For this review, take the finished solid that the model builds, in its own axes (mm). A direction names the side the tool comes from. Give positions to 0.01 mm unless a question says otherwise; leave off trailing zeros. Loops run counter-clockwise (first coordinate to the right, second up) from the corner with the lowest first, then second, coordinate; pieces in that order, holes last. Notation, with made-up numbers: (10, 55) - (18, 55) arc R30 ccw to (18, 83) - close; hole circle Ø3 at (45.25, -26.5). An arc over 180 degrees is marked (long way). Answer as CSV lines item,"result".
from build123d import *

# Parameters (mm, degrees)
SKETCH1_W           = 130
SKETCH1_H           = 50
BOSS_EXTRUDE1_DEPTH = 5
SKETCH2_W           = 130
SKETCH2_H           = 5
BOSS_EXTRUDE2_DEPTH = 32
SKETCH3_R           = 3
SKETCH3_W           = 5
SKETCH3_H           = 10
CUT_EXTRUDE1_DEPTH  = 10
FILLET1_R           = 5
CUT_EXTRUDE2_REACH  = 88.597
SKETCH4_R           = 3.15
SKETCH4_R_2         = 2.15


with BuildPart() as part:
    # Sketch1 → Boss-Extrude1 (new body)
    with BuildSketch(Plane(origin=(0, 0, 0), x_dir=(1, 0, 0), z_dir=(0, 1, 0))):
        Rectangle(SKETCH1_W, SKETCH1_H)
    extrude(amount=BOSS_EXTRUDE1_DEPTH)

    # Sketch2 → Boss-Extrude2 (add)
    with BuildSketch(Plane(origin=(0, 0, -25), x_dir=(-1, 0, 0), z_dir=(0, 0, -1))):
        with Locations((0, 2.5)):
            Rectangle(SKETCH2_W, SKETCH2_H)
    extrude(amount=BOSS_EXTRUDE2_DEPTH)

    # Sketch3 → Cut-Extrude1 (cut)
    with BuildSketch(Plane(origin=(0, 5, 0), x_dir=(1, 0, 0), z_dir=(0, 1, 0))):
        with Locations(Location((-57.5, 31.5, 0), (0, 0, 270))):
            Circle(SKETCH3_R)
        with Locations(Location((57.5, 31.5, 0), (0, 0, 270))):
            Circle(SKETCH3_R)
        with Locations((57.5, 44)):
            Rectangle(SKETCH3_W, SKETCH3_H)
        with Locations((-57.5, 19)):
            Rectangle(SKETCH3_W, SKETCH3_H)
        with Locations((-57.5, 44)):
            Rectangle(SKETCH3_W, SKETCH3_H)
        with Locations((57.5, 19)):
            Rectangle(SKETCH3_W, SKETCH3_H)
    extrude(amount=-CUT_EXTRUDE1_DEPTH, mode=Mode.SUBTRACT)

    # Fillet1
    fillet1_edges = [part.edges().sort_by_distance(p)[0] for p in [
        (65, 2.5, -57),
        (-65, 2.5, -57),
        (65, 2.5, 25),
        (-65, 2.5, 25),
    ]]
    fillet(fillet1_edges, radius=FILLET1_R)

    # Sketch4 → Cut-Extrude2 (cut, up to next)
    with BuildSketch(Plane(origin=(0, 5, 0), x_dir=(1, 0, 0), z_dir=(0, 1, 0)), mode=Mode.PRIVATE) as cut_extrude2_sk1:
        with Locations(Location((0, -0.5, 0), (0, 0, 270))):
            Circle(SKETCH4_R)
    cut_extrude2_tool1 = extrude(cut_extrude2_sk1.sketch, amount=-CUT_EXTRUDE2_REACH, mode=Mode.PRIVATE) & part.part
    # Sketch4 → Cut-Extrude2 (cut, up to next)
    with BuildSketch(Plane(origin=(0, 5, 0), x_dir=(1, 0, 0), z_dir=(0, 1, 0)), mode=Mode.PRIVATE) as cut_extrude2_sk2:
        with Locations(Location((25.4, 43.55, 0), (0, 0, 270))):
            Circle(SKETCH4_R_2)
    cut_extrude2_tool2 = extrude(cut_extrude2_sk2.sketch, amount=-CUT_EXTRUDE2_REACH, mode=Mode.PRIVATE) & part.part
    # Sketch4 → Cut-Extrude2 (cut, up to next)
    with BuildSketch(Plane(origin=(0, 5, 0), x_dir=(1, 0, 0), z_dir=(0, 1, 0)), mode=Mode.PRIVATE) as cut_extrude2_sk3:
        with Locations(Location((-25.4, 43.55, 0), (0, 0, 270))):
            Circle(SKETCH4_R_2)
    cut_extrude2_tool3 = extrude(cut_extrude2_sk3.sketch, amount=-CUT_EXTRUDE2_REACH, mode=Mode.PRIVATE) & part.part
    # Sketch4 → Cut-Extrude2 (cut, up to next)
    with BuildSketch(Plane(origin=(0, 5, 0), x_dir=(1, 0, 0), z_dir=(0, 1, 0)), mode=Mode.PRIVATE) as cut_extrude2_sk4:
        with Locations(Location((-12.7, 43.55, 0), (0, 0, 270))):
            Circle(SKETCH4_R_2)
    cut_extrude2_tool4 = extrude(cut_extrude2_sk4.sketch, amount=-CUT_EXTRUDE2_REACH, mode=Mode.PRIVATE) & part.part
    # Sketch4 → Cut-Extrude2 (cut, up to next)
    with BuildSketch(Plane(origin=(0, 5, 0), x_dir=(1, 0, 0), z_dir=(0, 1, 0)), mode=Mode.PRIVATE) as cut_extrude2_sk5:
        with Locations(Location((12.7, 43.55, 0), (0, 0, 270))):
            Circle(SKETCH4_R_2)
    cut_extrude2_tool5 = extrude(cut_extrude2_sk5.sketch, amount=-CUT_EXTRUDE2_REACH, mode=Mode.PRIVATE) & part.part
    # Sketch4 → Cut-Extrude2 (cut, up to next)
    with BuildSketch(Plane(origin=(0, 5, 0), x_dir=(1, 0, 0), z_dir=(0, 1, 0)), mode=Mode.PRIVATE) as cut_extrude2_sk6:
        with Locations(Location((0, 43.55, 0), (0, 0, 270))):
            Circle(SKETCH4_R_2)
    cut_extrude2_tool6 = extrude(cut_extrude2_sk6.sketch, amount=-CUT_EXTRUDE2_REACH, mode=Mode.PRIVATE) & part.part
    add(cut_extrude2_tool1.solids().sort_by_distance((0, 5, 0.5))[0], mode=Mode.SUBTRACT)
    add(cut_extrude2_tool2.solids().sort_by_distance((25.4, 5, -43.55))[0], mode=Mode.SUBTRACT)
    add(cut_extrude2_tool3.solids().sort_by_distance((-25.4, 5, -43.55))[0], mode=Mode.SUBTRACT)
    add(cut_extrude2_tool4.solids().sort_by_distance((-12.7, 5, -43.55))[0], mode=Mode.SUBTRACT)
    add(cut_extrude2_tool5.solids().sort_by_distance((12.7, 5, -43.55))[0], mode=Mode.SUBTRACT)
    add(cut_extrude2_tool6.solids().sort_by_distance((0, 5, -43.55))[0], mode=Mode.SUBTRACT)


solid = part.part
1) Insertion check: P1, Ø3.5, axis at x = -25.4, z = -43.55, coming from the +Y side. The pin has a flat end and moves straight along its axis. Give the tip position at first contact, or say it passes through.
From the geometry:
P1,"passes through"
2) Draft analysis for pull direction X (two halves, no side actions). For faces 1 (the flat face through (-1, 2, 25)), 2 (the cylindrical face through (64, 3, 23)), 3 (the cylindrical face through (-63, 3, 24)), 4 (the cylindrical face through (-1.917, 2.535, -2)), state which applies: pulls with the +X half, pulls with the -X half, needs draft (parallel to the pull), parting line crosses it, or undercut.
From the geometry:
face 1,"needs draft"
face 2,"pulls with the +X half"
face 3,"pulls with the -X half"
face 4,"undercut"
3) Consider section B-B on x = -25.4. Write out the cut boundary in (y, z), and give its area (4 significant figures).
From the geometry:
outline,"(0, -57) - (5, -57) - (5, -45.7) - (0, -45.7) - close; (0, -41.4) - (5, -41.4) - (5, 25) - (0, 25) - close"
area,"388.5 mm^2"
4) Consider section C-C on z = 0.5. Write out the cut boundary in (x, y), and give its area (4 significant figures).
From the geometry:
outline,"(-65, 0) - (-3.15, 0) - (-3.15, 5) - (-65, 5) - close; (3.15, 0) - (65, 0) - (65, 5) - (3.15, 5) - close"
area,"618.5 mm^2"
5) Machinability: for faces 5 (the flat face through (1, 5, -15)), 6 (the flat face through (57, 3, -39)), which of the approach directions +Z, -Z, +X, -X, +Y, -Y give a long, thin tool a straight path to every point of the face, cutting with its end or side? Answer none if there is none.
From the geometry:
face 5,"+Z, -Z, +X, -X, +Y"
face 6,"+Y, -Y"
6) Consider section D-D on y = 1.45. Count the separate pieces of the cut face and the enclosed holes in it, and give its area (3 significant figures).
From the geometry:
separate pieces,"1"
enclosed holes,"12"
area,"10,300 mm^2"
7) Wall thickness on line 1 (X direction, y = 0.5, z = -16); line 2 (Z direction, x = 13, y = 2.5); line 3 (X direction, y = 1.95, z = -1.5): over which ranges is each line inside the solid? List them lowest first. Write a range as from..to.
From the geometry:
line 1,"x = -65..-60, -55..55, 60..65"
line 2,"z = -57..-45.68, -41.42..25"
line 3,"x = -65..-2.43, 2.43..65"
8) Consider section A-A on z = -31.5. Write out the cut boundary in (x, y), and give its area (3 significant figures).
From the geometry:
outline,"(-65, 0) - (-60.5, 0) - (-60.5, 5) - (-65, 5) - close; (-54.5, 0) - (54.5, 0) - (54.5, 5) - (-54.5, 5) - close; (60.5, 0) - (65, 0) - (65, 5) - (60.5, 5) - close"
area,"590 mm^2"
